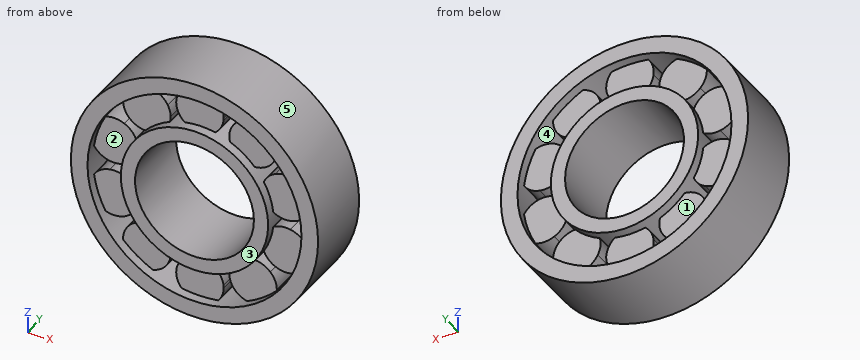
```python
from build123d import *

# Parameters (mm, degrees)
F2_R     = 26
F2_R_2   = 22.5
F3_DEPTH = 15
F1_R     = 15.5
F1_R_2   = 12.5
F4_DEPTH = 15
F6_DEPTH = 5.5


with BuildPart() as f3:
    # F2 (on Front) → F3 (new body)
    with BuildSketch(Plane.XZ):
        Circle(F2_R)
        Circle(F2_R_2, mode=Mode.SUBTRACT)
    extrude(amount=F3_DEPTH)



with BuildPart() as f4:
    # F1 (on Front) → F4 (new body)
    with BuildSketch(Plane.XZ):
        Circle(F1_R)
        Circle(F1_R_2, mode=Mode.SUBTRACT)
    extrude(amount=F4_DEPTH)


with BuildPart() as f3_1:
    add(f3.part)

    add(f4.part)  # F6 merges F4
    # F5 (on offset) → F6 (join, symmetric)
    with BuildSketch(Plane.XZ.offset(7.5)):
        with BuildLine():
            ThreePointArc((-18.97603, 0.954084), (-18.070074, 5.871323), (-15.912727, 10.381961))
            ThreePointArc((-15.912727, 10.381961), (-22.825356, 7.416408), (-18.97603, 0.954084))
        make_face()
        with BuildLine():
            ThreePointArc((-13.070074, 5.871323), (-13.840019, 8.53715), (-15.912727, 10.381961))
            ThreePointArc((-15.912727, 10.381961), (-18.070074, 5.871323), (-18.97603, 0.954084))
            ThreePointArc((-18.97603, 0.954084), (-14.870838, 2.028812), (-13.070074, 5.871323))
        make_face()
        with BuildLine():
            ThreePointArc((-18.97603, -0.954084), (-22.825356, -7.416408), (-15.912727, -10.381961))
            ThreePointArc((-15.912727, -10.381961), (-18.070074, -5.871323), (-18.97603, -0.954084))
        make_face()
        with BuildLine():
            ThreePointArc((-18.97603, -0.954084), (-18.070074, -5.871323), (-15.912727, -10.381961))
            ThreePointArc((-15.912727, -10.381961), (-13.840019, -8.53715), (-13.070074, -5.871323))
            ThreePointArc((-13.070074, -5.871323), (-14.870838, -2.028812), (-18.97603, -0.954084))
        make_face()
        with BuildLine():
            ThreePointArc((-14.791135, -11.925701), (-14.106846, -19.416408), (-6.771303, -17.752449))
            ThreePointArc((-6.771303, -17.752449), (-11.16792, -15.371323), (-14.791135, -11.925701))
        make_face()
        with BuildLine():
            ThreePointArc((-14.791135, -11.925701), (-11.16792, -15.371323), (-6.771303, -17.752449))
            ThreePointArc((-6.771303, -17.752449), (-6.321112, -16.599516), (-6.16792, -15.371323))
            ThreePointArc((-6.16792, -15.371323), (-9.312667, -10.72826), (-14.791135, -11.925701))
        make_face()
        with BuildLine():
            ThreePointArc((5, -19), (4.98912, -18.670335), (4.956528, -18.342105))
            ThreePointArc((4.956528, -18.342105), (0, -19), (-4.956528, -18.342105))
            ThreePointArc((-4.956528, -18.342105), (-0.329665, -23.98912), (5, -19))
        make_face()
        with BuildLine():
            ThreePointArc((-4.956528, -18.342105), (0, -19), (4.956528, -18.342105))
            ThreePointArc((4.956528, -18.342105), (0, -14), (-4.956528, -18.342105))
        make_face()
        with BuildLine():
            ThreePointArc((6.771303, -17.752449), (11.16792, -15.371323), (14.791135, -11.925701))
            ThreePointArc((14.791135, -11.925701), (8.228994, -11.326238), (6.771303, -17.752449))
        make_face()
        with BuildLine():
            ThreePointArc((16.16792, -15.371323), (15.810983, -13.51607), (14.791135, -11.925701))
            ThreePointArc((14.791135, -11.925701), (11.16792, -15.371323), (6.771303, -17.752449))
            ThreePointArc((6.771303, -17.752449), (12.396113, -20.21813), (16.16792, -15.371323))
        make_face()
        with BuildLine():
            ThreePointArc((15.912727, -10.381961), (18.070074, -5.871323), (18.97603, -0.954084))
            ThreePointArc((18.97603, -0.954084), (13.314791, -4.326238), (15.912727, -10.381961))
        make_face()
        with BuildLine():
            ThreePointArc((23.070074, -5.871323), (21.912585, -2.672087), (18.97603, -0.954084))
            ThreePointArc((18.97603, -0.954084), (18.070074, -5.871323), (15.912727, -10.381961))
            ThreePointArc((15.912727, -10.381961), (20.735901, -10.101378), (23.070074, -5.871323))
        make_face()
        with BuildLine():
            ThreePointArc((15.912727, 10.381961), (13.314791, 4.326238), (18.97603, 0.954084))
            ThreePointArc((18.97603, 0.954084), (18.070074, 5.871323), (15.912727, 10.381961))
        make_face()
        with BuildLine():
            ThreePointArc((15.912727, 10.381961), (18.070074, 5.871323), (18.97603, 0.954084))
            ThreePointArc((18.97603, 0.954084), (21.912585, 2.672087), (23.070074, 5.871323))
            ThreePointArc((23.070074, 5.871323), (20.735901, 10.101378), (15.912727, 10.381961))
        make_face()
        with BuildLine():
            ThreePointArc((6.771303, 17.752449), (8.228994, 11.326238), (14.791135, 11.925701))
            ThreePointArc((14.791135, 11.925701), (11.16792, 15.371323), (6.771303, 17.752449))
        make_face()
        with BuildLine():
            ThreePointArc((6.771303, 17.752449), (11.16792, 15.371323), (14.791135, 11.925701))
            ThreePointArc((14.791135, 11.925701), (15.810983, 13.51607), (16.16792, 15.371323))
            ThreePointArc((16.16792, 15.371323), (12.396113, 20.21813), (6.771303, 17.752449))
        make_face()
        with BuildLine():
            ThreePointArc((-4.956528, 18.342105), (0, 19), (4.956528, 18.342105))
            ThreePointArc((4.956528, 18.342105), (4.98912, 18.670335), (5, 19))
            ThreePointArc((5, 19), (-0.329665, 23.98912), (-4.956528, 18.342105))
        make_face()
        with BuildLine():
            ThreePointArc((-4.956528, 18.342105), (0, 14), (4.956528, 18.342105))
            ThreePointArc((4.956528, 18.342105), (0, 19), (-4.956528, 18.342105))
        make_face()
        with BuildLine():
            ThreePointArc((-6.16792, 15.371323), (-6.321112, 16.599516), (-6.771303, 17.752449))
            ThreePointArc((-6.771303, 17.752449), (-11.16792, 15.371323), (-14.791135, 11.925701))
            ThreePointArc((-14.791135, 11.925701), (-9.312667, 10.72826), (-6.16792, 15.371323))
        make_face()
        with BuildLine():
            ThreePointArc((-14.791135, 11.925701), (-11.16792, 15.371323), (-6.771303, 17.752449))
            ThreePointArc((-6.771303, 17.752449), (-14.106846, 19.416408), (-14.791135, 11.925701))
        make_face()
    extrude(amount=F6_DEPTH, both=True)


solid = f3_1.part
```
Design review of the part built by this model. Coordinates are the model's own, in mm. Face numbers are marked on the shaded views. A direction names the side the tool comes from. Coordinates: 2 decimals unless noted, no trailing zeros. Order: outer loops, then holes, each group sorted by start corner. A loop starts at its lowest first (then second) coordinate and runs counter-clockwise, first axis right, second up.
1) Take a section at D-D, the plane y = -14. Give the boundary of the cut face in (x, z), and give its area (3 significant figures).
2) Take a section at B-B, the plane z = 0. Give the boundary of the cut face in (x, y).
3) For the marked faces 1 and 2, list the 3-axis set-ups (+Z, -Z, +X, -X, +Y, -Y) from which the entire face can be reached by the end or side of a thin tool; tool diameter is ignored.
4) Clearance check with flat-ended pins moving along their axes: pin 1 (3 mm diameter, centred on x = 9, z = 15, fed in from -Y); pin 2 (4.5 mm diameter, centred on x = -17.5, z = -8.5, fed in from +Y); pin 3 (8 mm diameter, centred on y = -2.5, z = -1, fed in from +X); pin 4 (3 mm diameter, centred on x = -5.5, y = -7, fed in from -Z). State where each tip first meets the part, or that it passes through.
5) Take a section at C-C, the plane x = -9. Give the boundary of the cut face in (y, z).
6) Take a section at A-A, the plane x = 0. Give the boundary of the cut face in (y, z).
7) Mouldability with a two-part tool opening along X and no side actions: class the marked faces 3, 4 and 5 as +X half, -X half, draft (parallel to the pull), parting line (faces both ways), or undercut.
8) Wall thickness on line 1 along Z through (x, y) = (-14, -13.5); line 2 along Z through (x, y) = (0, -7); line 3 along Z through (x, y) = (-4.5, -2.75): over which ranges is each line inside the solid? List them lowest first.
Returned:
1. outline: circle Ø52 at (0, 0); circle Ø31 at (0, 0); hole circle Ø45 at (0, 0); hole circle Ø25 at (0, 0)
1. area: 797 mm2
2. outline: (-26, -15) - (-22.5, -15) - (-22.5, 0) - (-26, 0) - close; (-15.5, -15) - (-12.5, -15) - (-12.5, 0) - (-15.5, 0) - close; (12.5, -15) - (15.5, -15) - (15.5, 0) - (12.5, 0) - close; (22.5, -15) - (26, -15) - (26, 0) - (22.5, 0) - close
3. face 1: +Y
3. face 2: -Y
4. pin 1: stops at y = -13
4. pin 2: stops at y = -2
4. pin 3: stops at x = 26
4. pin 4: stops at z = -25.69
5. outline: (-15, -24.39) - (0, -24.39) - (0, -20.62) - (-15, -20.62) - close; (-15, -12.62) - (-13, -12.62) - (-13, -19.88) - (-2, -19.88) - (-2, -12.62) - (0, -12.62) - (0, -8.67) - (-15, -8.67) - close; (-15, 8.67) - (0, 8.67) - (0, 12.62) - (-2, 12.62) - (-2, 19.88) - (-13, 19.88) - (-13, 12.62) - (-15, 12.62) - close; (-15, 20.62) - (0, 20.62) - (0, 24.39) - (-15, 24.39) - close
6. outline: (-15, -26) - (0, -26) - (0, -22.5) - (-2, -22.5) - (-2, -15.5) - (0, -15.5) - (0, -12.5) - (-15, -12.5) - (-15, -15.5) - (-13, -15.5) - (-13, -22.5) - (-15, -22.5) - close; (-15, 12.5) - (0, 12.5) - (0, 15.5) - (-2, 15.5) - (-2, 22.5) - (0, 22.5) - (0, 26) - (-15, 26) - (-15, 22.5) - (-13, 22.5) - (-13, 15.5) - (-15, 15.5) - close
7. face 3: draft
7. face 4: undercut
7. face 5: parting line
8. line 1: z = -21.91 to -17.61, -6.65 to 6.65, 17.61 to 21.91
8. line 2: z = -26 to -12.5, 12.5 to 26
8. line 3: z = -25.61 to -22.05, -21.18 to -16.82, -14.83 to -11.66, 11.66 to 14.83, 16.82 to 21.18, 22.05 to 25.61
